Build history of the part. All positions in model axes, mm. Give positions to 0.01 mm unless a question says otherwise; leave off trailing zeros. Loops run counter-clockwise (first coordinate to the right, second up) from the corner with the lowest first, then second, coordinate; pieces in that order, holes last. Notation, with made-up numbers: (40.25, 56.5) -> (91.25, 56.5) arc R36 cw to (91.25, 91.5) -> close; hole circle Ø11 at (0.25, 79.5). An arc over 180 degrees is marked (long way). Answer in a Markdown table with one row per item. Add a question column.
from build123d import *

# Parameters (mm, degrees)
F1_DEPTH = 15


with BuildPart() as f1:
    # F0 (on Front) → F1 (new body)
    with BuildSketch(Plane.XZ):
        with BuildLine():
            Line((23.603925, 11.403642), (21.103925, 11.403642))
            ThreePointArc((21.103925, 11.403642), (18.174993, 4.332574), (11.103925, 1.403642))
            ThreePointArc((11.103925, 1.403642), (4.032858, 4.332574), (1.103925, 11.403642))
            Line((1.103925, 11.403642), (-1.396075, 11.403642))
            Line((-1.396075, 11.403642), (-1.396075, -8.596358))
            Line((-1.396075, -8.596358), (23.603925, -8.596358))
            Line((23.603925, -8.596358), (23.603925, 11.403642))
        make_face()
    extrude(amount=F1_DEPTH)


solid = f1.part
(1) Saw through at D-D, the plane x = 3.5. List the corners of the cut face in (y, z), then the cut area to 3 significant figures.
(2) Wall check: line 1 along X through (y, z) = (-9.25, 5.75); line 2 along X through (y, z) = (-3.25, 8.5); line 3 along Z through (x, y) = (7.5, -8.75). Give the ranges that are in metal, low to high. Write a range as from..to.
(3) Saw through at C-C, the plane x = 19.75. List the corners of the cut face in (y, z), then the cut area to 3 significant figures.
(4) Saw through at B-B, the plane y = -3.75. List the corners of the cut face in (x, z).
(5) Saw through at A-A, the plane z = 5.5. List the corners of the cut face in (x, y), then the cut area to 3 significant figures.
Worked answers:
| question | item | result |
|---|---|---|
| 1 | outline | (-15, -8.6) -> (0, -8.6) -> (0, 4.91) -> (-15, 4.91) -> close |
| 1 | area | 203 mm^2 |
| 2 | line 1 | -1.4..2.86, 19.35..23.6 |
| 2 | line 2 | -1.4..1.53, 20.67..23.6 |
| 2 | line 3 | -8.6..2.08 |
| 3 | outline | (-15, -8.6) -> (0, -8.6) -> (0, 6.38) -> (-15, 6.38) -> close |
| 3 | area | 225 mm^2 |
| 4 | outline | (-1.4, -8.6) -> (23.6, -8.6) -> (23.6, 11.4) -> (21.1, 11.4) arc R10 cw to (11.1, 1.4) arc R10 cw to (1.1, 11.4) -> (-1.4, 11.4) -> close |
| 5 | outline | (-1.4, -15) -> (3.03, -15) -> (3.03, 0) -> (-1.4, 0) -> close; (19.18, -15) -> (23.6, -15) -> (23.6, 0) -> (19.18, 0) -> close |
| 5 | area | 133 mm^2 |
